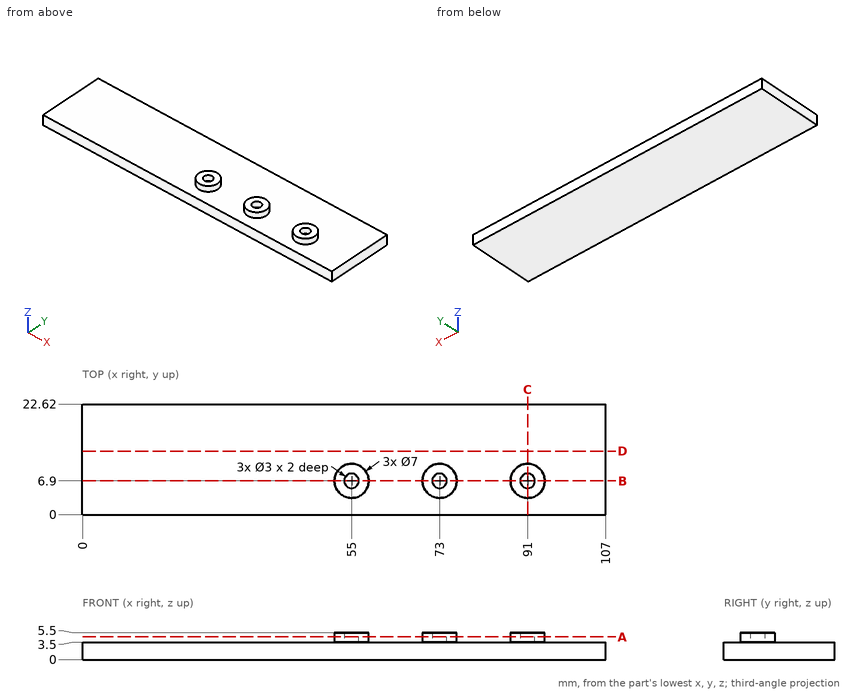
Check sheet for the drawn part. Datum: minimum x, y, z corner. Units: mm. Coordinates: 2 decimals unless noted, no trailing zeros. Loops run counter-clockwise (first coordinate to the right, second up) from the corner with the lowest first, then second, coordinate; pieces in that order, holes last. Notation, with made-up numbers: M 56,9 L 104,9 A19 ccw 104,34 Z; hole C -32.75,37.5 d6. An arc over 180 degrees is marked long. Answer as a JSON object with one key per item and string values.
1. Sectioned sample at A-A on z = 4.65. Record the cut outline in (x, y), and give its area (3 significant figures).
Outcome:
{"outline": "C 55,6.9 d7; C 73,6.9 d7; C 91,6.9 d7; hole C 55,6.9 d3; hole C 73,6.9 d3; hole C 91,6.9 d3", "area": "94.2 mm²"}
2. Scan lines: L1, parallel to Y at x = 73, z = 4.25; L2, parallel to X at y = 9.75, z = 4.2; L3, parallel to Z at x = 15.5, y = 2.5. Record each from-to range of solid material in increasing order. Write a range as from..to.
Outcome:
{"L1": "3.4..5.4, 8.4..10.4", "L2": "52.97..57.03, 70.97..75.03, 88.97..93.03", "L3": "0..3.5"}
3. Depth check by flat-ended pin: P1, Ø1.8, axis at x = 55, y = 6.9, coming from the -Z side; P2, Ø4, axis at x = 20.5, y = 6.5, coming from the +Z side. Enter the tip coordinate at first touch or a pass-through.
Outcome:
{"P1": "z = 0", "P2": "z = 3.5"}
4. Sectioned sample at B-B on y = 6.9. Record the cut outline in (x, z), and give its area (4 significant figures).
Outcome:
{"outline": "M 0,0 L 107,0 L 107,3.5 L 94.5,3.5 L 94.5,5.5 L 92.5,5.5 L 92.5,3.5 L 89.5,3.5 L 89.5,5.5 L 87.5,5.5 L 87.5,3.5 L 76.5,3.5 L 76.5,5.5 L 74.5,5.5 L 74.5,3.5 L 71.5,3.5 L 71.5,5.5 L 69.5,5.5 L 69.5,3.5 L 58.5,3.5 L 58.5,5.5 L 56.5,5.5 L 56.5,3.5 L 53.5,3.5 L 53.5,5.5 L 51.5,5.5 L 51.5,3.5 L 0,3.5 Z", "area": "398.5 mm²"}
5. Sectioned sample at C-C on x = 91. Record the cut outline in (y, z).
Outcome:
{"outline": "M 0,0 L 22.62,0 L 22.62,3.5 L 10.4,3.5 L 10.4,5.5 L 8.4,5.5 L 8.4,3.5 L 5.4,3.5 L 5.4,5.5 L 3.4,5.5 L 3.4,3.5 L 0,3.5 Z"}
6. Sectioned sample at D-D on y = 13. Record the cut outline in (x, z), and give its area (4 significant figures).
Outcome:
{"outline": "M 0,0 L 107,0 L 107,3.5 L 0,3.5 Z", "area": "374.5 mm²"}
